Here's how the part is built. I have some questions about the finished solid (model axes, mm). Face numbers are marked on the shaded views. A direction names the side the tool comes from. Round coordinates to 2 decimals unless told otherwise and drop trailing zeros. Answer as CSV lines item,"result".
from build123d import *

# Parameters (mm, degrees)
F0_W     = 55
F0_H     = 5
F0_W_2   = 10
F0_H_2   = 10
F3_DEPTH = 100
F4_DEPTH = 30
F6_DEPTH = 20


with BuildPart() as f2:
    # F1 (on Front) → F2 (revolve)
    with BuildSketch(Plane.XZ):
        with BuildLine():
            Line((-50, 0), (0, 0))
            Line((0, 0), (0, 50))
            ThreePointArc((0, 50), (-35.355339, 35.355339), (-50, 0))
        make_face()
    revolve(axis=Axis((0, 0, 25), (0, 0, 1)))

    # F0 (on Top) → F3 (cut)
    with BuildSketch(Plane.XY):
        with Locations((0, -19.5)):
            Rectangle(F0_W, F0_H)
        with Locations((0, 19.5)):
            Rectangle(F0_W, F0_H)
        Rectangle(F0_W_2, F0_H_2)
    extrude(amount=F3_DEPTH, mode=Mode.SUBTRACT)

    # F0 (on Top) → F4 (cut)
    with BuildSketch(Plane.XY):
        Polygon((27.5, 17), (-27.5, 17), (-27.5, 5), (-27.5, -5), (-27.5, -17), (27.5, -17), (27.5, -5), (27.5, 5), align=None)
        Rectangle(F0_W_2, F0_H_2, mode=Mode.SUBTRACT)
    extrude(amount=F4_DEPTH, mode=Mode.SUBTRACT)

    # F5 (on Top) → F6 (cut)
    with BuildSketch(Plane.XY):
        with BuildLine():
            ThreePointArc((-27.5, 5), (-32.5, 0), (-27.5, -5))
            Line((-27.5, -5), (-27.5, 5))
        make_face()
        with BuildLine():
            Line((27.5, 5), (27.5, -5))
            ThreePointArc((27.5, -5), (32.5, 0), (27.5, 5))
        make_face()
    extrude(amount=F6_DEPTH, mode=Mode.SUBTRACT)


solid = f2.part
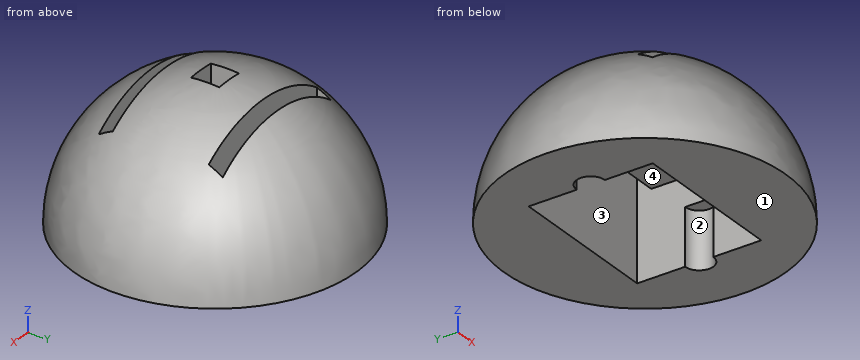
Item 1: For the marked faces 3 and 4, which set-ups out of +Z, -Z, +X, -X, +Y, -Y let a thin tool reach every point of the face, with its end or its side?
Results found:
face 3,"+Z, -Z"
face 4,"-Z"
Item 2: I need wall thicknesses on L1, parallel to Y at x = 3.5, z = 32; L2, parallel to Y at x = 9, z = 28.5; L3, parallel to Y at x = 16, z = 22.5. Which ranges of each line are inside material? Lowest first, please.
Results found:
L1,"y = -38.26 to -22, -17 to -5, 5 to 17, 22 to 38.26"
L2,"y = -40.08 to -22, 22 to 40.08"
L3,"y = -41.69 to -22, 22 to 41.69"
Item 3: Suppose I cut it at A-A, the plane z = 41. State how many separate pieces and enclosed holes the cut face has, then the cut area to 3 significant figures.
Results found:
separate pieces,"3"
enclosed holes,"1"
area,"2,060 mm²"
Item 4: If we mould it in two halves opening along Y, with no side actions, what happens to the marked faces 1 and 2? For each: pulls with the +Y half, pulls with the -Y half, needs draft (parallel to the pull), parting line crosses it, or undercut.
Results found:
face 1,"needs draft"
face 2,"undercut"
Item 5: Will these pins go through, and if not, where does the flat tip stop? pin 1 (5.5 mm diameter, centred on x = 30.5, y = -0.5, fed in from -Z); pin 2 (1.5 mm diameter, centred on x = 20, z = 5, fed in from +Y); pin 3 (3 mm diameter, centred on x = 1, z = 40, fed in from -Y); pin 4 (6 mm diameter, centred on x = 17, z = 29, fed in from -Y).
Results found:
pin 1,"stops at z = 0"
pin 2,"stops at y = 45.88"
pin 3,"stops at y = -31.89"
pin 4,"stops at y = -39.53"
